Check sheet for the modelled part. Datum: model origin and axes. Units: mm. Round coordinates to 2 decimals unless told otherwise and drop trailing zeros. Order: outer loops, then holes, each group sorted by start corner. A loop starts at its lowest first (then second) coordinate and runs counter-clockwise, first axis right, second up.
Autodesk Inventor part; units mm, degrees
ref_plane "YZ Plane" through (0, 0, 0) normal (1, 0, 0) x (0, 1, 0)
ref_plane "XZ Plane" through (0, 0, 0) normal (0, 1, 0) x (-1, 0, 0)
ref_plane "XY Plane" through (0, 0, 0) normal (0, 0, 1) x (1, 0, 0)
sketch "Esboço1" plane through (0, 0, 0) normal (0, 0, 1) x (1, 0, 0)
  line L0 (-26.8932, 18.2034) -> (37.1068, 18.2034)
  line L1 (37.1068, 18.2034) -> (37.1068, -32.7966)
  line L2 (37.1068, -32.7966) -> (-26.8932, -32.7966)
  line L3 (-26.8932, -32.7966) -> (-26.8932, 18.2034)
  circle A0 centre (-20.2432, 11.2034) radius 3
  circle A1 centre (-20.2432, -25.7966) radius 3
  circle A2 centre (30.4568, -25.7966) radius 3
  circle A3 centre (30.4568, 11.2034) radius 3
  dimension "d9" = 64
  dimension "d10" = 51
  dimension "d15" = 6
  dimension "d16" = 6
  dimension "d17" = 6
  dimension "d18" = 6
  dimension "d26" = 50.7
  dimension "d27" = 37
  dimension "d28" = 50.7
  dimension "d29" = 37
  dimension "d31" = 6.65
  dimension "d33" = 6.65
  dimension "d34" = 7
  dimension "d36" = 7
  dimension "d37" = 7
  dimension "d38" = 7
extrude "Extrusão1" add sketch "Esboço1" along normal blind 1
chamfer "Chanfro1" distance 1 angle 45 4 edges at (-23.2432, -25.7966, 1) (-23.2432, 11.2034, 1) (27.4568, 11.2034, 1) (27.4568, -25.7966, 1)
fillet "Arredondamento2" radius 7 4 edges at (-26.8932, -32.7966, 0.5) (37.1068, -32.7966, 0.5) (37.1068, 18.2034, 0.5) (-26.8932, 18.2034, 0.5)
properties part number "alguma parte da guitarra"
1) Sectioned sample at A-A on z = 0.4. Record the cut outline in (x, y), and give its area (3 significant figures).
2) Sectioned sample at B-B on y = -27. Count the separate pieces of the cut face and the enclosed holes in it, and give its area (3 significant figures).
3) Gauge pin test, flat end, axial feed: pin 1 (5.5 mm diameter, centred on x = -20.24, y = 11.2, fed in from +Z). Record the tip position at first contact, or that the pin passes through.
4) Scan lines: line 1 (Y direction, x = -17.5, z = 0.2); line 2 (Y direction, x = 29, z = 0.4); line 3 (X direction, y = 14, z = 0.5). Record each from-to range of solid material in increasing order.
Values found:
1. outline: (-26.89, -25.8) arc R7 ccw to (-19.89, -32.8) - (30.11, -32.8) arc R7 ccw to (37.11, -25.8) - (37.11, 11.2) arc R7 ccw to (30.11, 18.2) - (-19.89, 18.2) arc R7 ccw to (-26.89, 11.2) - close; hole circle Ø6.8 at (-20.24, -25.8); hole circle Ø6.8 at (-20.24, 11.2); hole circle Ø6.8 at (30.46, -25.8); hole circle Ø6.8 at (30.46, 11.2)
1. area: 3,080 mm2
2. separate pieces: 3
2. enclosed holes: 0
2. area: 50.7 mm2
3. pin 1: passes through
4. line 1: y = -32.8 to -27.44, -24.15 to 9.56, 12.85 to 18.2
4. line 2: y = -32.8 to -28.87, -22.73 to 8.13, 14.27 to 18.2
4. line 3: x = -26.31 to -22.35, -18.14 to 28.35, 32.56 to 36.52
